from build123d import *

# Parameters (mm, degrees)
SKETCH_1_R      = 1.5
EXTRUDE_1_DEPTH = 19
EXTRUDE_START   = 6.5
SKETCH_2_R      = 1.5
EXTRUDE_2_DEPTH = 6.5
SKETCH_3_R      = 1.5
EXTRUDE_3_DEPTH = 3
SKETCH_4_R      = 2.5
SKETCH_4_R_2    = 1.5
EXTRUDE_4_DEPTH = 0.5


with BuildPart() as part:
    # 草图1 → 凸台-拉伸1 (new body)
    with BuildSketch(Plane(origin=(0, 0, 0), x_dir=(1, 0, 0), z_dir=(0, 1, 0))):
        with Locations(Location((0, 0, 0), (0, 0, 270))):
            Circle(SKETCH_1_R)
    extrude(amount=EXTRUDE_1_DEPTH)

    # 草图2 → 凸台-拉伸2 (add)
    with BuildSketch(Plane(origin=(0, 13, 0), x_dir=(-1, 0, 0), z_dir=(0, -1, 0)).offset(EXTRUDE_START)):
        with BuildLine():
            Line((0.911921049, 1.78), (-0.911921049, 1.78))
            ThreePointArc((-0.911921049, 1.78), (0, -2), (0.911921049, 1.78))
        make_face()
        with Locations(Location((0, 0, 0), (0, 0, 90))):
            Circle(SKETCH_2_R, mode=Mode.SUBTRACT)
    extrude(amount=-EXTRUDE_2_DEPTH)

    # 草图3 → 凸台-拉伸3 (add)
    with BuildSketch(Plane(origin=(0, 13, 0), x_dir=(1, 0, 0), z_dir=(0, 1, 0))):
        with BuildLine():
            Line((0.91625301, 1.777774007), (-1.022249701, 1.719012958))
            ThreePointArc((-1.022249701, 1.719012958), (0.060597358, -1.999081779), (0.91625301, 1.777774007))
        make_face()
        with Locations(Location((0, 0, 0), (0, 0, 90))):
            Circle(SKETCH_3_R, mode=Mode.SUBTRACT)
    extrude(amount=EXTRUDE_3_DEPTH)

    # 草图4 → 凸台-拉伸4 (add)
    with BuildSketch(Plane(origin=(0, 13, 0), x_dir=(1, 0, 0), z_dir=(0, 1, 0))):
        with Locations(Location((0, 0, 0), (0, 0, 270))):
            Circle(SKETCH_4_R)
        with Locations(Location((0, 0, 0), (0, 0, 90))):
            Circle(SKETCH_4_R_2, mode=Mode.SUBTRACT)
    extrude(amount=EXTRUDE_4_DEPTH)


solid = part.part
Input: part model. Units: mm. Frame: model coordinates. A direction names the side the tool comes from. Coordinates: 2 decimals unless noted, no trailing zeros. Loops run counter-clockwise (first coordinate to the right, second up) from the corner with the lowest first, then second, coordinate; pieces in that order, holes last.
Q1. Material intervals for line 1 (X direction, y = 12, z = 0); line 2 (Y direction, x = 1.7, z = 0.1); line 3 (X direction, y = 17.75, z = 0.05), sorted ascending.
Q2. Cut plane D-D (z = 2.25). Output: boundary loops of the cut face in (x, y).
Q3. Contact query for flat-ended pins moving along their axis: pin 1 (1 mm diameter, centred on x = 1.5, z = -1.5, fed in from +Y); pin 2 (2 mm diameter, centred on x = -0.5, y = 10, fed in from -Z); pin 3 (1 mm diameter, centred on y = 3, z = 0, fed in from -X). Output: stop coordinate, or through.
Q4. Set-up query: faces 1 (the face through (0.45, 3.2, 1.43)), 2 (the face through (0, 10, -1.78)), 3 (the face through (0, 19, 0)), 4 (the face through (-2.44, 13.25, -0.54)), 5 (the face through (0, 15, 2)). Return all of +Z, -Z, +X, -X, +Y, -Y with unobstructed straight access to the full face (end or side cutting, diameter ignored); none if empty.
Q5. Cut plane B-B (x = 0). Output: boundary loops of the cut face in (y, z).
Q6. Cut plane A-A (z = 0). Output: boundary loops of the cut face in (x, y), then the cut area to 3 significant figures.
Q7. Cut plane C-C (y = 12.5). Output: boundary loops of the cut face in (x, z), then the cut area to 3 significant figures.
Working result:
1. line 1: x = -2 to 2
1. line 2: y = 6.5 to 16
1. line 3: x = -1.5 to 1.5
2. outline: (-1.09, 13) - (1.09, 13) - (1.09, 13.5) - (-1.09, 13.5) - close
3. pin 1: stops at y = 16
3. pin 2: stops at z = -1.78
3. pin 3: stops at x = -1.5
4. face 1: -Y
4. face 2: -Z, +X, -X, -Y
4. face 3: +Z, -Z, +X, -X, +Y
4. face 4: +Y, -Y
4. face 5: +Y
5. outline: (0, -1.5) - (6.5, -1.5) - (6.5, -1.78) - (13, -1.78) - (13, -2.5) - (13.5, -2.5) - (13.5, -1.75) - (16, -1.75) - (16, -1.5) - (19, -1.5) - (19, 1.5) - (16, 1.5) - (16, 2) - (13.5, 2) - (13.5, 2.5) - (13, 2.5) - (13, 2) - (6.5, 2) - (6.5, 1.5) - (0, 1.5) - close
6. outline: (-2.5, 13) - (-2, 13) - (-2, 6.5) - (-1.5, 6.5) - (-1.5, 0) - (1.5, 0) - (1.5, 6.5) - (2, 6.5) - (2, 13) - (2.5, 13) - (2.5, 13.5) - (2, 13.5) - (2, 16) - (1.5, 16) - (1.5, 19) - (-1.5, 19) - (-1.5, 16) - (-2, 16) - (-2, 13.5) - (-2.5, 13.5) - close
6. area: 67.0 mm2
7. outline: (-0.91, -1.78) - (0.91, -1.78) arc R2 ccw (long way) to start
7. area: 12.3 mm2
